```python
from build123d import *

# Parameters (mm, degrees)
EXTRUDE1_DEPTH                 = 10
EXTRUDE2_DEPTH                 = 7
SKETCH5_W                      = 26
SKETCH5_H                      = 15
EXTRUDE3_DEPTH                 = 7
SKETCH16_W                     = 6
SKETCH16_H                     = 22
SKETCH16_H_2                   = 10.7
EXTRUDE8_DEPTH                 = 7
F_8_CLEARANCE_HOLE1_AT_2_COUNT = 2
F_8_CLEARANCE_HOLE1_AT_2_PITCH = 15
F_8_CLEARANCE_HOLE2_AT_2_COUNT = 2
F_8_CLEARANCE_HOLE2_AT_2_PITCH = 15
EXTRUDE6_DEPTH                 = 4
SKETCH15_W                     = 12
SKETCH15_H                     = 170.1
EXTRUDE7_DEPTH                 = 7
FILLET1_R                      = 3.175
CHAMFER1_SIZE                  = 0.5
CHAMFER2_SIZE                  = 0.3
FILLET4_R                      = 3
FILLET3_R                      = 0.5


with BuildPart() as part:
    # Sketch1 → Extrude1 (new body)
    with BuildSketch(Plane(origin=(0, 0, 0), x_dir=(1, 0, 0), z_dir=(0, 1, 0))):
        Polygon((-126.1, 2198), (-165.1, 2198), (-165.1, 1998.9), (-145.1, 1998.9), (-145.1, 1988.2), (-145.1, 1987.6), (-145.1, 1976.9), (-165.1, 1976.9), (-165.1, 1382.9), (-145.1, 1382.9), (-145.1, 1372.2), (-126.1, 1372.2), align=None)
    extrude(amount=-EXTRUDE1_DEPTH)

    # Sketch4 → Extrude2 (cut)
    with BuildSketch(Plane.XZ.offset(10)):
        Polygon((-139.1, -1372.2), (-129.1, -1372.2), (-129.1, -2198), (-139.1, -2198), (-139.1, -1946.9), (-165.1, -1946.9), (-165.1, -1412.9), (-139.1, -1412.9), align=None)
    extrude(amount=-EXTRUDE2_DEPTH, mode=Mode.SUBTRACT)

    # Sketch5 → Extrude3 (cut)
    with BuildSketch(Plane.XZ.offset(10)):
        with Locations((-152.1, -1390.4)):
            Rectangle(SKETCH5_W, SKETCH5_H)
        with Locations((-152.1, -2006.4)):
            Rectangle(SKETCH5_W, SKETCH5_H)
        with Locations((-152.1, -1969.4)):
            Rectangle(SKETCH5_W, SKETCH5_H)
    extrude(amount=-EXTRUDE3_DEPTH, mode=Mode.SUBTRACT)

    # Sketch16 → Extrude8 (cut)
    with BuildSketch(Plane.XZ.offset(10)):
        with Locations((-142.1, -1987.9)):
            Rectangle(SKETCH16_W, SKETCH16_H)
        with Locations((-142.1, -1377.55)):
            Rectangle(SKETCH16_W, SKETCH16_H_2)
    extrude(amount=-EXTRUDE8_DEPTH, mode=Mode.SUBTRACT)

    # Sketch9 → 1/8 (0.125) Diameter Hole1 (revolve, cut)
    with BuildSketch(Plane(origin=(-152.6, -3, -2004.9), x_dir=(0, 0, -1), z_dir=(1, 0, 0))):
        Polygon((0, 0), (0, 3), (2.2479, 3), (1.6129, 2.365), (1.6129, 0.635), (2.2479, 0), align=None)
    revolve(axis=Axis((-152.6, -9.35, -2004.9), (0, 1, 0)), mode=Mode.SUBTRACT)

    # Sketch17 → 1/8 (0.125) Diameter Hole2 (revolve, cut)
    with BuildSketch(Plane(origin=(-152.6, -3, -1970.9), x_dir=(0, 0, -1), z_dir=(1, 0, 0))):
        Polygon((0, 0), (0, 3), (2.2479, 3), (1.6129, 2.365), (1.6129, 0.635), (2.2479, 0), align=None)
    revolve(axis=Axis((-152.6, -9.35, -1970.9), (0, 1, 0)), mode=Mode.SUBTRACT)

    # Sketch10 → #8 Clearance Hole1 (revolve, cut)
    with BuildSketch(Plane(origin=(-160.1, -3, -1970.9), x_dir=(0, 0, -1), z_dir=(1, 0, 0))):
        Polygon((0, 0), (0, 3), (3.0861, 3), (2.45745, 2.37135), (2.45745, 0.635), (3.09245, 0), align=None)
    f_8_clearance_hole1 = revolve(axis=Axis((-160.1, -9.35, -1970.9), (0, 1, 0)), mode=Mode.SUBTRACT)

    # #8 Clearance Hole1 at 2: #8 Clearance Hole1 ×2
    with Locations(*[(i * F_8_CLEARANCE_HOLE1_AT_2_PITCH, 0, 0) for i in range(1, F_8_CLEARANCE_HOLE1_AT_2_COUNT)]):
        add(f_8_clearance_hole1, mode=Mode.SUBTRACT)

    # Sketch14 → #8 Clearance Hole2 (revolve, cut)
    with BuildSketch(Plane(origin=(-160.1, -3, -2004.9), x_dir=(0, 0, -1), z_dir=(1, 0, 0))):
        Polygon((0, 0), (0, 3), (3.0861, 3), (2.45745, 2.37135), (2.45745, 0.635), (3.09245, 0), align=None)
    f_8_clearance_hole2 = revolve(axis=Axis((-160.1, -9.35, -2004.9), (0, 1, 0)), mode=Mode.SUBTRACT)

    # #8 Clearance Hole2 at 2: #8 Clearance Hole2 ×2
    with Locations(*[(i * F_8_CLEARANCE_HOLE2_AT_2_PITCH, 0, 0) for i in range(1, F_8_CLEARANCE_HOLE2_AT_2_COUNT)]):
        add(f_8_clearance_hole2, mode=Mode.SUBTRACT)

    # Sketch12 → Extrude6 (cut, through all)
    with BuildSketch(Plane.XZ.offset(3)):
        with BuildLine():
            Line((-154.251, -1387.9), (-154.251, -1389.9))
            ThreePointArc((-154.251, -1389.9), (-152.6, -1391.551), (-150.949, -1389.9))
            Line((-150.949, -1389.9), (-150.949, -1387.9))
            ThreePointArc((-150.949, -1387.9), (-152.6, -1386.249), (-154.251, -1387.9))
        make_face()
        with BuildLine():
            Line((-162.85, -1389.9), (-162.85, -1387.9))
            ThreePointArc((-162.85, -1387.9), (-160.1, -1385.15), (-157.35, -1387.9))
            Line((-157.35, -1387.9), (-157.35, -1389.9))
            ThreePointArc((-157.35, -1389.9), (-160.1, -1392.65), (-162.85, -1389.9))
        make_face()
        with BuildLine():
            Line((-147.85, -1389.9), (-147.85, -1387.9))
            ThreePointArc((-147.85, -1387.9), (-145.1, -1385.15), (-142.35, -1387.9))
            Line((-142.35, -1387.9), (-142.35, -1389.9))
            ThreePointArc((-142.35, -1389.9), (-145.1, -1392.65), (-147.85, -1389.9))
        make_face()
    extrude(amount=-EXTRUDE6_DEPTH, mode=Mode.SUBTRACT)

    # Sketch15 → Extrude7 (cut)
    with BuildSketch(Plane.XZ.offset(10)):
        with Locations((-152.1, -2105.95)):
            Rectangle(SKETCH15_W, SKETCH15_H)
    extrude(amount=-EXTRUDE7_DEPTH, mode=Mode.SUBTRACT)

    # Fillet1
    fillet1_edges = [part.edges().sort_by_distance(p)[0] for p in [
        (-146.1, -6.5, -2020.9),
        (-158.1, -6.5, -2020.9),
        (-158.1, -6.5, -2191),
        (-146.1, -6.5, -2191),
    ]]
    fillet(fillet1_edges, radius=FILLET1_R)

    # Chamfer1
    chamfer1_edges = [part.edges().sort_by_distance(p)[0] for p in [
        (-129.1, -6.5, -2198),
        (-126.1, -5, -2198),
        (-139.1, -6.5, -2198),
        (-134.1, -3, -2198),
        (-145.6, 0, -2198),
        (-165.1, -5, -2198),
        (-152.1, -10, -2198),
        (-145.1, -1.5, -1372.2),
        (-137.1, -3, -1372.2),
        (-135.6, 0, -1372.2),
        (-126.1, -5, -1372.2),
        (-127.6, -10, -1372.2),
        (-129.1, -6.5, -1372.2),
    ]]
    chamfer(chamfer1_edges, length=CHAMFER1_SIZE)

    # Chamfer2
    chamfer2_edges = [part.edges().sort_by_distance(p)[0] for p in [
        (-152.6, 0, -1386.249),
        (-150.949, 0, -1388.9),
        (-152.6, 0, -1391.551),
        (-154.251, 0, -1388.9),
        (-152.6, -3, -1386.249),
        (-154.251, -3, -1388.9),
        (-152.6, -3, -1391.551),
        (-150.949, -3, -1388.9),
        (-160.1, 0, -1385.15),
        (-157.35, 0, -1388.9),
        (-160.1, 0, -1392.65),
        (-162.85, 0, -1388.9),
        (-160.1, -3, -1385.15),
        (-162.85, -3, -1388.9),
        (-160.1, -3, -1392.65),
        (-157.35, -3, -1388.9),
        (-145.1, 0, -1385.15),
        (-142.35, 0, -1388.9),
        (-145.1, 0, -1392.65),
        (-147.85, 0, -1388.9),
        (-145.1, -3, -1385.15),
        (-147.85, -3, -1388.9),
        (-145.1, -3, -1392.65),
        (-142.35, -3, -1388.9),
    ]]
    chamfer(chamfer2_edges, length=CHAMFER2_SIZE)

    # Fillet4
    fillet4_edges = [part.edges().sort_by_distance(p)[0] for p in [
        (-139.1, -6.5, -1412.9),
        (-139.1, -6.5, -1946.9),
        (-139.1, -6.5, -1397.9),
        (-139.1, -6.5, -2013.9),
        (-139.1, -6.5, -1961.9),
    ]]
    fillet(fillet4_edges, radius=FILLET4_R)

    # Fillet3
    fillet3_edges = [part.edges().sort_by_distance(p)[0] for p in [
        (-146.1, -3, -2105.95),
        (-152.1, -3, -2191),
        (-152.1, -3, -2020.9),
        (-158.1, -3, -2105.95),
        (-147.02993597, -3, -2021.82993597),
        (-157.17006403, -3, -2021.82993597),
        (-157.17006403, -3, -2190.07006403),
        (-147.02993597, -3, -2190.07006403),
        (-129.1, -3, -1785.1),
        (-139.1, -3, -2107.2),
        (-153.6, -3, -1961.9),
        (-139.1, -3, -1954.4),
        (-153.6, -3, -1412.9),
        (-139.1, -3, -1405.4),
        (-139.978679656, -3, -2014.778679656),
        (-139.978679656, -3, -1961.021320344),
        (-139.978679656, -3, -1947.778679656),
        (-139.978679656, -3, -1412.021320344),
        (-139.978679656, -3, -1398.778679656),
        (-153.6, -3, -1946.9),
        (-153.6, -3, -1397.9),
        (-153.6, -3, -2013.9),
    ]]
    fillet(fillet3_edges, radius=FILLET3_R)


solid = part.part
```
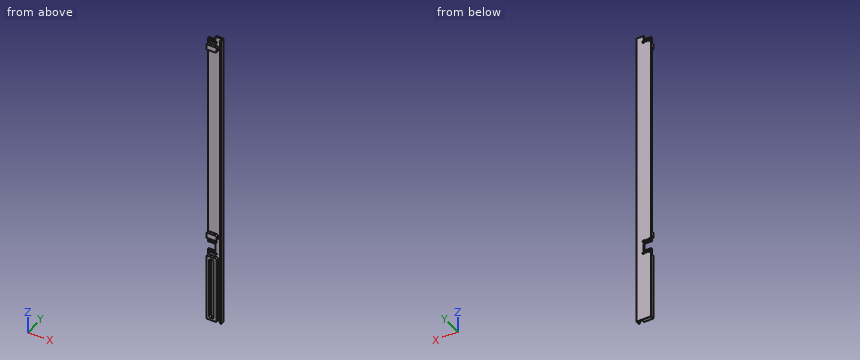
Here's how the part is built. I have some questions about the finished solid (model axes, mm). Give positions to 0.01 mm unless a question says otherwise; leave off trailing zeros. Write each loop counter-clockwise with the first axis right and the second up, starting at its lowest first coordinate (ties: lowest second). Pieces come first, ordered by that corner, then holes. Notation, with made-up numbers: M 72.5,13 L 114.5,13 A20 cw 114.5,51 Z; hole C -2,49.5 d10. An arc over 180 degrees is marked long. Put each result on its own line as item: value. Start each with the question number.
Item 1: If we section it at C-C, the plane z = -2058: Write out the boundary of the cut face in (x, y), then the cut area to 3 significant figures.
Item 2: If we section it at A-A, the plane z = -1473: Write out the boundary of the cut face in (x, y).
Item 3: If we section it at B-B, the plane y = -7.5: Count the separate pieces of the cut face and the enclosed holes in it, then the cut area to 3 significant figures.
Item 4: Will these pins go through, and if not, where does the flat tip stop? pin 1 (5 mm diameter, centred on x = -149.5, y = -8, fed in from +Z); pin 2 (6 mm diameter, centred on x = -140.5, z = -1617, fed in from -Y); pin 3 (6 mm diameter, centred on x = -158.5, y = -3, fed in from +Z).
Item 5: I need wall thicknesses on L1, parallel to Z at x = -152.6, y = -1.2; L2, parallel to Z at x = -142.5, y = -9; L3, parallel to Z at x = -160.1, y = -1.95. Which ranges of each line are inside material? Lowest first, please. Write a range as from..to.
Values:
1. outline: M -165.1,-10 L -158.1,-10 L -158.1,-3.5 A0.5 cw -157.6,-3 L -146.6,-3 A0.5 cw -146.1,-3.5 L -146.1,-10 L -139.1,-10 L -139.1,-3.5 A0.5 cw -138.6,-3 L -129.6,-3 A0.5 cw -129.1,-3.5 L -129.1,-10 L -126.1,-10 L -126.1,0 L -165.1,0 Z
1. area: 236 mm²
2. outline: M -165.1,-3 L -129.6,-3 A0.5 cw -129.1,-3.5 L -129.1,-10 L -126.1,-10 L -126.1,0 L -165.1,0 Z
3. separate pieces: 4
3. enclosed holes: 1
3. area: 6,000 mm²
4. pin 1: z = -1397.9
4. pin 2: y = -3
4. pin 3: z = -1382.9
5. L1: -2198..-2006.51, -2003.29..-1998.9, -1976.9..-1972.51, -1969.29..-1391.55, -1386.25..-1382.9
5. L2: -2198..-2013.9, -1961.9..-1946.9, -1412.9..-1397.9
5. L3: -2198..-2007.36, -2002.44..-1998.9, -1976.9..-1973.36, -1968.44..-1392.65, -1385.15..-1382.9
